Verification items for the finished model (mm, model axes). Round coordinates to 2 decimals unless told otherwise and drop trailing zeros. Write each loop counter-clockwise with the first axis right and the second up, starting at its lowest first coordinate (ties: lowest second). Pieces come first, ordered by that corner, then holes. Notation, with made-up numbers: (62.25, 80.25) - (115.25, 80.25) arc R21 ccw to (115.25, 109.25) - close; hole circle Ø3 at (-21, -24). An arc over 180 degrees is marked (long way). Answer as a JSON object with one key per item and string values.
Autodesk Inventor part; units mm, degrees
ref_plane "YZ Plane" through (0, 0, 0) normal (1, 0, 0) x (0, 1, 0)
ref_plane "XZ Plane" through (0, 0, 0) normal (0, 1, 0) x (-1, 0, 0)
ref_plane "XY Plane" through (0, 0, 0) normal (0, 0, 1) x (1, 0, 0)
sketch "Skizze2" plane through (0, 0, 0) normal (0, 1, 0) x (-1, 0, 0)
  circle A0 centre (0, 0) radius 75
  line L0 (-102.5, -200) -> (102.5, -200)
  line L1 (102.5, -200) -> (102.5, 200)
  line L2 (102.5, 200) -> (-102.5, 200)
  line L3 (-102.5, 200) -> (-102.5, -200)
  line L4 (-102.5, -200) -> (102.5, 200) construction
  line L5 (102.5, -200) -> (-102.5, 200) construction
  dimension "d8" = 150
  dimension "d9" = 205
  dimension "d10" = 400
extrude "Extrusion1" add sketch "Skizze2" along normal blind 15
sketch "Skizze3" plane through (0, 0, 0) normal (0, -1, 0) x (1, 0, 0)
  line L0 (-90, -190) -> (90, -190)
  line L1 (90, -190) -> (90, 190)
  line L2 (90, 190) -> (-90, 190)
  line L3 (-90, 190) -> (-90, -190)
  line L4 (-90, -190) -> (90, 190) construction
  line L5 (90, -190) -> (-90, 190) construction
  point P0 (0, 0)
  dimension "d13" = 180
  dimension "d14" = 380
hole "Bohrung1" at (90, 0, -190) at (-90, 0, -190) at (-90, 0, 190) at (90, 0, 190) direction (0, 1, 0) diameter 4.917 end through all
sketch "Skizze4" plane through (-102.5, 0, 200) normal (0, 0, 1) x (1, 0, 0)
  line L0 (0, 0) -> (0, 15)
  line L1 (0, 0) -> (205, 0)
  line L2 (205, 0) -> (205, 15)
  point P0 (102.5, 0)
  point P1 (40, 7.5)
  point P2 (165, 7.5)
  point P3 (76, 7.5)
  point P4 (129, 7.5)
  dimension "d23" = 40
  dimension "d24" = 7.5
  dimension "d25" = 7.5
  dimension "d44" = 36
  dimension "d45" = 36
  dimension "d46" = 7.5
  dimension "d47" = 7.5
  dimension "d48" = 40
sketch "Skizze5" plane through (102.5, 0, -200) normal (0, 0, -1) x (-1, 0, 0)
  line L0 (205, 0) -> (205, 15)
  line L1 (0, 0) -> (205, 0)
  line L2 (0, 0) -> (0, 15)
  point P0 (102.5, 0)
  point P1 (40, 7.5)
  point P2 (165, 7.5)
  point P3 (76, 7.5)
  point P4 (129, 7.5)
  dimension "d27" = 40
  dimension "d28" = 7.5
  dimension "d29" = 7.5
  dimension "d49" = 7.5
  dimension "d50" = 7.5
  dimension "d51" = 36
  dimension "d52" = 36
  dimension "d53" = 40
hole "Bohrung4" at (62.5, 7.5, -200) at (26.5, 7.5, -200) at (-26.5, 7.5, -200) at (-62.5, 7.5, -200) direction (0, 0, 1) diameter 4.134 depth 14.2 tip angle 118
hole "Bohrung5" at (-62.5, 7.5, 200) at (62.5, 7.5, 200) at (-26.5, 7.5, 200) at (26.5, 7.5, 200) direction (0, 0, -1) diameter 4.134 depth 14.2 tip angle 118
sketch "Skizze6" plane through (0, 0, 0) normal (0, -1, 0) x (1, 0, 0)
  line L0 (99, 200) -> (99, -200)
  line L1 (102.5, 200) -> (102.5, -200)
  line L2 (96.5, 200) -> (96.5, -200)
  line L3 (-99, -200) -> (-99, 200)
  line L4 (-96.5, -200) -> (-96.5, 200)
  line L5 (102.5, -200) -> (-102.5, -200)
  line L6 (96.5, -200) -> (99, -200)
  line L7 (-96.5, -200) -> (-99, -200)
  line L8 (-102.5, 200) -> (102.5, 200)
  line L9 (-96.5, 200) -> (-99, 200)
  line L10 (99, 200) -> (96.5, 200)
  line L11 (-102.5, -200) -> (-102.5, 200)
  point P0 (0, 0)
  point P1 (96.5, 200)
  dimension "d68" = 2.5
  dimension "d70" = 2.5
  dimension "d84" = 198
  dimension "d85" = 99
extrude "Extrusion2" cut sketch "Skizze6" against normal blind 2.5 contours L0 L5 L2 L8 | L4 L5 L3 L8
sketch "Skizze7" plane through (0, 0, 0) normal (0, -1, 0) x (1, 0, 0)
  line L0 (-80, -20) -> (80, -20)
  line L1 (80, -20) -> (80, 20)
  line L2 (80, 20) -> (-80, 20)
  line L3 (-80, 20) -> (-80, -20)
  line L4 (-80, -20) -> (80, 20) construction
  line L5 (80, -20) -> (-80, 20) construction
  point P0 (0, 0)
  dimension "d74" = 160
  dimension "d75" = 40
hole "Bohrung6" at (-80, 0, 20) at (-80, 0, -20) at (80, 0, -20) at (80, 0, 20) direction (0, 1, 0) diameter 4.134 end through all
equation "\"d70\" = d68"
properties part number "Grundplatte1.0"
Q1. Release check for a two-part mould opening along X. For faces 1 (the cylindrical face through (9.764, 7.395, -74.362)), 2 (the flat face through (1, 7, -200)), 3 (the flat face through (102.5, 7, 3)) record: released by +X, released by -X, zero draft, split by the parting line, or undercut.
Geometry check:
{"face 1": "undercut", "face 2": "zero draft", "face 3": "released by +X"}
Q2. Material ranges on line 1 along X through (y, z) = (7.5, 196.5); line 2 along Z through (x, y) = (80, 9.25); line 3 along Z through (x, y) = (90, 4.5), recorded low to high. Write a range as [from, to].
Geometry check:
{"line 1": "x = [-102.5, -64.57], [-60.43, -28.57], [-24.43, 24.43], [28.57, 60.43], [64.57, 102.5]", "line 2": "z = [-200, -22.07], [-17.93, 17.93], [22.07, 200]", "line 3": "z = [-200, -192.46], [-187.54, 187.54], [192.46, 200]"}
Q3. Section check A-A, the plane z = 0. Record the cut outline in (x, y), then the cut area to 4 significant figures.
Geometry check:
{"outline": "(-102.5, 0) - (-99, 0) - (-99, 2.5) - (-96.5, 2.5) - (-96.5, 0) - (-75, 0) - (-75, 15) - (-102.5, 15) - close; (75, 0) - (96.5, 0) - (96.5, 2.5) - (99, 2.5) - (99, 0) - (102.5, 0) - (102.5, 15) - (75, 15) - close", "area": "812.5 mm2"}
Q4. Gauge pin test, flat end, axial feed: P1, Ø3.5, axis at x = -62.5, y = 7.5, coming from the +Z side. Record the tip position at first contact, or that the pin passes through.
Geometry check:
{"P1": "stops at z = 185.61"}
